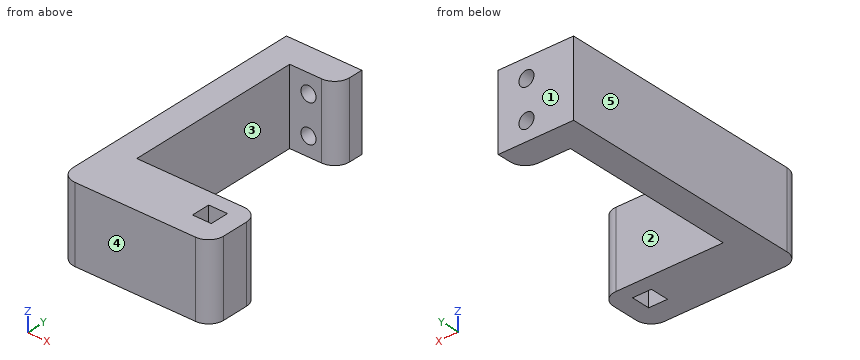
from build123d import *

# Parameters (mm, degrees)
BOSS_EXTRUDE1_DEPTH = 25.4
SKETCH2_W           = 12.7
SKETCH2_H           = 12.7
CUT_EXTRUDE1_DEPTH  = 50.8
SKETCH3_R           = 5.072330543
CUT_EXTRUDE2_DEPTH  = 50.8


with BuildPart() as part:
    # Sketch1 → Boss-Extrude1 (new, symmetric)
    with BuildSketch(Plane.XY):
        with BuildLine():
            Line((10.16, 0), (91.44, 0))
            ThreePointArc((91.44, 0), (98.624204897, 2.975795103), (101.6, 10.16))
            Line((101.6, 10.16), (101.6, 27.94))
            ThreePointArc((101.6, 27.94), (98.624204897, 35.124204897), (91.44, 38.1))
            Line((91.44, 38.1), (19.05, 38.1))
            Line((19.05, 38.1), (19.05, 158.129767442))
            Line((19.05, 158.129767442), (40.64, 158.129767442))
            ThreePointArc((40.64, 158.129767442), (47.824204897, 161.105562545), (50.8, 168.289767442))
            Line((50.8, 168.289767442), (50.8, 177.8))
            Line((50.8, 177.8), (0, 177.8))
            Line((0, 177.8), (0, 10.16))
            ThreePointArc((0, 10.16), (2.975795103, 2.975795103), (10.16, 0))
        make_face()
    extrude(amount=BOSS_EXTRUDE1_DEPTH, both=True)

    # Sketch2 → Cut-Extrude1 (cut)
    with BuildSketch(Plane.XY.offset(25.4)):
        with Locations((82.55, 21.59)):
            Rectangle(SKETCH2_W, SKETCH2_H)
    extrude(amount=-CUT_EXTRUDE1_DEPTH, mode=Mode.SUBTRACT)

    # Sketch3 → Cut-Extrude2 (cut)
    with BuildSketch(Plane.XZ.offset(-158.129767442)):
        with Locations(Location((31.75, 12.7, 0), (0, 0, 270))):
            Circle(SKETCH3_R)
        with Locations(Location((31.75, -12.7, 0), (0, 0, 270))):
            Circle(SKETCH3_R)
    extrude(amount=-CUT_EXTRUDE2_DEPTH, mode=Mode.SUBTRACT)


solid = part.part
CAD build for the part. Positions are in the model's coordinates, mm. Face numbers are marked on the shaded views. A direction names the side the tool comes from. Coordinates: 2 decimals unless noted, no trailing zeros. Loops run counter-clockwise (first coordinate to the right, second up) from the corner with the lowest first, then second, coordinate; pieces in that order, holes last. Notation, with made-up numbers: (-16.5, 29) - (2.5, 29) arc R17 ccw to (2.5, 58) - close; hole circle Ø6 at (82.25, 49.25). An arc over 180 degrees is marked (long way). Use one line per item in the form item = value. Start each with the question number.
1) Two-plate mould, pull along Y, no slides. Class the marked faces 3, 4 and 5: +Y half, -Y half, draft (parallel to the pull), parting line (faces both ways), or undercut.
2) Band-saw the part on D-D (x = 31.75). Give the cut face in (y, z).
3) Drill centre lines: L1, parallel to X at y = 170, z = -12.7; L2, parallel to Y at x = 30, z = 6.5; L3, parallel to Z at x = 31, y = 173. Where is each one in solid material? Low to high. Write a range as from..to.
4) Band-saw the part on A-A (z = 12.7). Give the cut face in (x, y).
5) Tool access for the marked faces 1 and 2: list every direction of +Z, -Z, +X, -X, +Y, -Y with a clear straight run to the whole face (end or side of a thin tool).
6) Band-saw the part on C-C (y = 25.5). Give the cut face in (x, z).
7) Band-saw the part on B-B (x = 85.5). Give the cut face in (y, z), and give its area (3 significant figures).
8) Flat gauge pins, fed straight in: pin 1 (6.5 mm diameter, centred on x = 84.5, z = 2, fed in from +Y); pin 2 (2 mm diameter, centred on y = 29.5, z = -7.5, fed in from +X); pin 3 (3 mm diameter, centred on y = 174.5, z = 9, fed in from +X). Where does each tip first touch, or does it go through?
Check values:
q1.face_3 = undercut
q1.face_4 = -Y half
q1.face_5 = draft
q2.outline = (0, -25.4) - (38.1, -25.4) - (38.1, 25.4) - (0, 25.4) - close; (158.13, -25.4) - (177.8, -25.4) - (177.8, -17.77) - (158.13, -17.77) - close; (158.13, -7.63) - (177.8, -7.63) - (177.8, 7.63) - (158.13, 7.63) - close; (158.13, 17.77) - (177.8, 17.77) - (177.8, 25.4) - (158.13, 25.4) - close
q3.L1 = 0..26.68, 36.82..50.8
q3.L2 = 0..38.1, 158.13..177.8
q3.L3 = -25.4..-17.72, -7.68..7.68, 17.72..25.4
q4.outline = (0, 10.16) arc R10.16 ccw to (10.16, 0) - (91.44, 0) arc R10.16 ccw to (101.6, 10.16) - (101.6, 27.94) arc R10.16 ccw to (91.44, 38.1) - (19.05, 38.1) - (19.05, 158.13) - (26.68, 158.13) - (26.68, 177.8) - (0, 177.8) - close; (36.82, 158.13) - (40.64, 158.13) arc R10.16 ccw to (50.8, 168.29) - (50.8, 177.8) - (36.82, 177.8) - close; hole (76.2, 15.24) - (88.9, 15.24) - (88.9, 27.94) - (76.2, 27.94) - close
q5.face_1 = +Z, -Z, +X, -X, +Y
q5.face_2 = +Z, -Z, +X
q6.outline = (0, -25.4) - (76.2, -25.4) - (76.2, 25.4) - (0, 25.4) - close; (88.9, -25.4) - (101.6, -25.4) - (101.6, 25.4) - (88.9, 25.4) - close
q7.outline = (0, -25.4) - (15.24, -25.4) - (15.24, 25.4) - (0, 25.4) - close; (27.94, -25.4) - (38.1, -25.4) - (38.1, 25.4) - (27.94, 25.4) - close
q7.area = 1,290 mm2
q8.pin_1 = 38.1
q8.pin_2 = 101.58
q8.pin_3 = 50.8
